```python
from build123d import *

# Parameters (mm, degrees)
F0_W     = 75
F0_H     = 75
F1_DEPTH = 10
F2_W     = 65
F2_H     = 65
F3_DEPTH = 10
F4_R     = 2.5
F5_DEPTH = 20.001


with BuildPart() as f1:
    # F0 (on Top) → F1 (new body)
    with BuildSketch(Plane.XY):
        Rectangle(F0_W, F0_H)
    extrude(amount=F1_DEPTH)

    # F2 (on face) → F3 (join)
    with BuildSketch(Plane.XY.offset(10)):
        Rectangle(F2_W, F2_H)
    extrude(amount=F3_DEPTH)

    # F4 (on face) → F5 (cut, through all)
    with BuildSketch(Plane.XY.offset(20)):
        with Locations((-25.5, 25.5)):
            Circle(F4_R)
        with Locations((25.5, 25.5)):
            Circle(F4_R)
        with Locations((25.5, -25.5)):
            Circle(F4_R)
        with Locations((-25.5, -25.5)):
            Circle(F4_R)
    extrude(amount=-F5_DEPTH, mode=Mode.SUBTRACT)


solid = f1.part
```
Here's how the part is built. I have some questions about the finished solid (model axes, mm). A direction names the side the tool comes from. Coordinates: 2 decimals unless noted, no trailing zeros. Order: outer loops, then holes, each group sorted by start corner. A loop starts at its lowest first (then second) coordinate and runs counter-clockwise, first axis right, second up. Notation, with made-up numbers: (34, 80) -> (93, 80) arc R28 ccw to (93, 98) -> close; hole circle Ø6 at (1, 84.5). An arc over 180 degrees is marked (long way). Return JSON: item names as keys, results as strings.
1) I'm going to push flat-ended pins straight in: P1, Ø3, axis at x = 1, z = 14.5, coming from the -Y side; P2, Ø2, axis at x = 11, z = 13, coming from the +Y side; P3, Ø8, axis at y = -15.5, z = 16.5, coming from the +X side. Where does each tip first touch, or does it pass through?
Conclusion:
{"P1": "stops at y = -32.5", "P2": "stops at y = 32.5", "P3": "stops at x = 32.5"}
2) If we section it at D-D on x = -9.5: List the corners of the cut face in (y, z) for me, plus the area to 3 significant figures.
Conclusion:
{"outline": "(-37.5, 0) -> (37.5, 0) -> (37.5, 10) -> (32.5, 10) -> (32.5, 20) -> (-32.5, 20) -> (-32.5, 10) -> (-37.5, 10) -> close", "area": "1,400 mm²"}
3) If we section it at C-C on z = 15.25: List the corners of the cut face in (x, y) for me.
Conclusion:
{"outline": "(-32.5, -32.5) -> (32.5, -32.5) -> (32.5, 32.5) -> (-32.5, 32.5) -> close; hole circle Ø5 at (-25.5, -25.5); hole circle Ø5 at (-25.5, 25.5); hole circle Ø5 at (25.5, -25.5); hole circle Ø5 at (25.5, 25.5)"}
4) If I drill on probe 1 along Y at (x, z) = (-25.5, 7.5); probe 2 along Y at (x, z) = (25.5, 13.75); probe 3 along Z at (x, y) = (33, 19.5), over which ranges is the centre line in solid material (lowest first)?
Conclusion:
{"probe 1": "y = -37.5 to -28, -23 to 23, 28 to 37.5", "probe 2": "y = -32.5 to -28, -23 to 23, 28 to 32.5", "probe 3": "z = 0 to 10"}
5) If we section it at A-A on y = 25.5: List the corners of the cut face in (x, z) for me.
Conclusion:
{"outline": "(-37.5, 0) -> (-28, 0) -> (-28, 20) -> (-32.5, 20) -> (-32.5, 10) -> (-37.5, 10) -> close; (-23, 0) -> (23, 0) -> (23, 20) -> (-23, 20) -> close; (28, 0) -> (37.5, 0) -> (37.5, 10) -> (32.5, 10) -> (32.5, 20) -> (28, 20) -> close"}
6) Thinking about a two-plate mould opening in X: for faces 1 (the flat face through (-1, 37.5, 5)), 2 (the cylindrical face through (25.17, -23.02, 10.14)), 3 (the flat face through (32.5, 0, 15)), which applies, +X half, -X half, draft (parallel to the pull), parting line (faces both ways), or undercut?
Conclusion:
{"face 1": "draft", "face 2": "undercut", "face 3": "+X half"}
7) On a 3-axis mill with a long thin cutter (end or side, diameter ignored), from which of +Z, -Z, +X, -X, +Y, -Y can I reach the whole of each face in a straight line? I mean faces 4 (the flat face through (0, 0, 20)), 5 (the flat face through (0, -32.5, 15)), 6 (the flat face through (0, 32.5, 15)), 7 (the flat face through (-32.5, 0, 15)). Say none if no direction works.
Conclusion:
{"face 4": "+Z, +X, -X, +Y, -Y", "face 5": "+Z, +X, -X, -Y", "face 6": "+Z, +X, -X, +Y", "face 7": "+Z, -X, +Y, -Y"}
